Answer from the drawing. Dimensions are ordinates in mm from the lowest x, y and z of the part. Give positions to 0.01 mm unless a question says otherwise; leave off trailing zeros. Order: outer loops, then holes, each group sorted by start corner. A loop starts at its lowest first (then second) coordinate and runs counter-clockwise, first axis right, second up. Notation, with made-up numbers: (69, -17.5) - (112, -17.5) arc R30 ccw to (112, 12.5) - close; hole circle Ø6 at (-21, 85). An arc over 180 degrees is marked (long way). Answer in a Markdown table with one row per item.
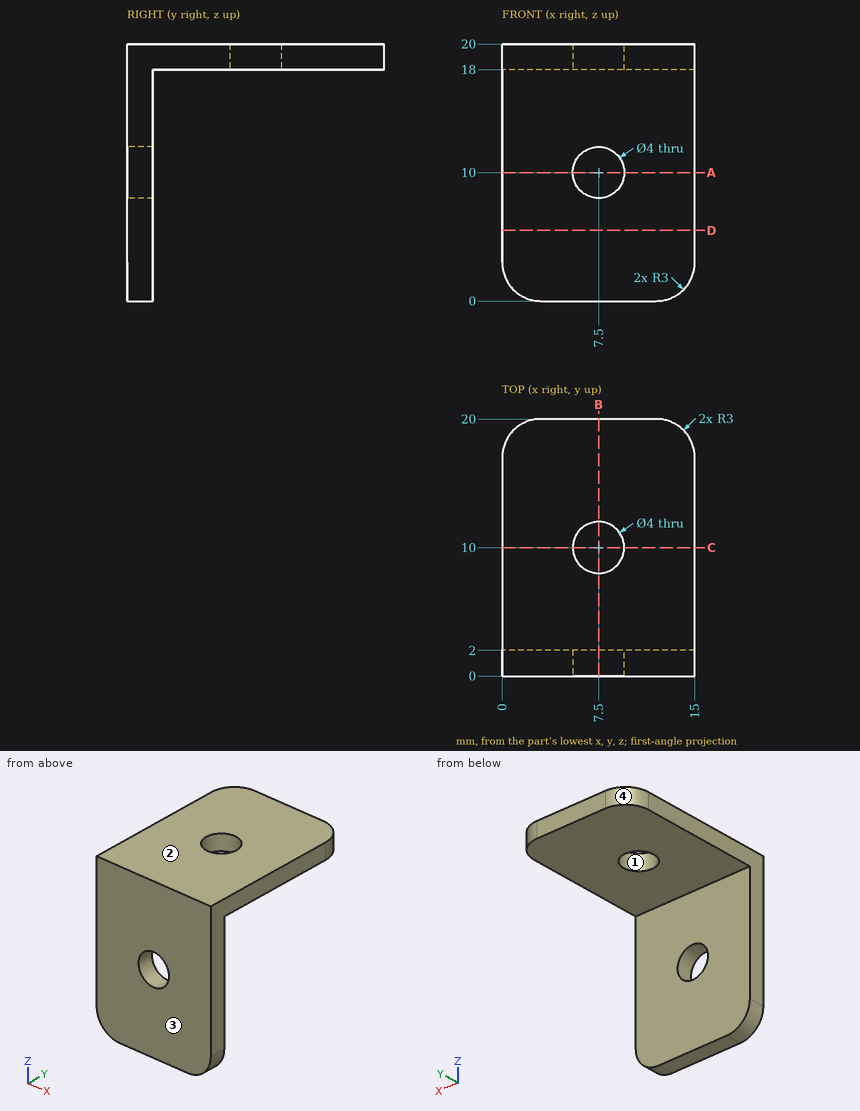
Item 1: Find section D-D on z = 5.5. Write down the section's boundary in (x, y).
Answer block:
| item | result |
|---|---|
| outline | (0, 0) - (15, 0) - (15, 2) - (0, 2) - close |
Item 2: Find section B-B on x = 7.5. Write down the section's boundary in (y, z), then the cut area to 3 significant figures.
Answer block:
| item | result |
|---|---|
| outline | (0, 0) - (2, 0) - (2, 8) - (0, 8) - close; (0, 12) - (2, 12) - (2, 18) - (8, 18) - (8, 20) - (0, 20) - close; (12, 18) - (20, 18) - (20, 20) - (12, 20) - close |
| area | 60.0 mm² |
Item 3: Consider line 1 (Y direction, x = 7.5, z = 19.55); line 2 (X direction, y = 1.4, z = 10). Determine where each line is inside the solid, lowest interval first.
Answer block:
| item | result |
|---|---|
| line 1 | 0 to 8, 12 to 20 |
| line 2 | 0 to 5.5, 9.5 to 15 |
Item 4: Find section A-A on z = 10. Write down the section's boundary in (x, y), then the cut area to 3 significant figures.
Answer block:
| item | result |
|---|---|
| outline | (0, 0) - (5.5, 0) - (5.5, 2) - (0, 2) - close; (9.5, 0) - (15, 0) - (15, 2) - (9.5, 2) - close |
| area | 22.0 mm² |
Item 5: Find section C-C on y = 10. Write down the section's boundary in (x, z).
Answer block:
| item | result |
|---|---|
| outline | (0, 18) - (5.5, 18) - (5.5, 20) - (0, 20) - close; (9.5, 18) - (15, 18) - (15, 20) - (9.5, 20) - close |
Item 6: Determine the mould class of the marked faces 1, 2, 3 and 4 for opening direction Y: pulls with the +Y half, pulls with the -Y half, needs draft (parallel to the pull), parting line crosses it, or undercut.
Answer block:
| item | result |
|---|---|
| face 1 | undercut |
| face 2 | needs draft |
| face 3 | pulls with the -Y half |
| face 4 | pulls with the +Y half |
Item 7: Each of these flat-tipped pins is pushed along its axis until it touches: P1, Ø2, axis at x = 11.5, y = 6.5, coming from the -Z side; P2, Ø6, axis at y = 16, z = 12.5, coming from the +X side; P3, Ø5, axis at x = 2.5, z = 6.5, coming from the +Y side. Where does it stop, or does it pass through?
Answer block:
| item | result |
|---|---|
| P1 | z = 18 |
| P2 | through |
| P3 | y = 2 |
